Can you work these out from the model? Positions are in its coordinate system, mm. A direction names the side the tool comes from. Coordinates: 2 decimals unless noted, no trailing zeros. Order: outer loops, then holes, each group sorted by start corner. A loop starts at its lowest first (then second) coordinate and runs counter-clockwise, first axis right, second up. Notation, with made-up numbers: (85.25, 10.25) -> (128.25, 10.25) arc R28 cw to (128.25, 38.25) -> close; hole circle Ø9 at (-21, 68.5). An arc over 180 degrees is marked (long way). Write item = value, one per line. Start each with the question number.
from build123d import *

# Parameters (mm, degrees)
BOSS_EXTRUDE1_DEPTH            = 9.525
CUT_EXTRUDE2_DEPTH             = 4
M3_CLEARANCE_HOLE1_D           = 3.2
M3_CLEARANCE_HOLE1_CSINK_D     = 3.45
M3_CLEARANCE_HOLE1_CSINK_ANGLE = 90
FILLET1_R                      = 1


with BuildPart() as part:
    # Sketch2 → Boss-Extrude1 (new body)
    with BuildSketch(Plane(origin=(0, 0, 0), x_dir=(0, 1, 0), z_dir=(0, 0, 1))):
        with BuildLine():
            Line((-9, 10), (9, 10))
            Line((9, 10), (50.45475081, -78.9))
            ThreePointArc((50.45475081, -78.9), (0, -93.653039883), (-50.45475081, -78.9))
            Line((-50.45475081, -78.9), (-9, 10))
        make_face()
    extrude(amount=BOSS_EXTRUDE1_DEPTH)

    # Sketch3 → Cut-Extrude2 (cut)
    with BuildSketch(Plane(origin=(0, 0, 0), x_dir=(1, 0, 0), z_dir=(0, 0, -1))):
        with BuildLine():
            Line((-10, -4.5), (-10, 4.5))
            Line((-10, 4.5), (0, 4.5))
            ThreePointArc((0, 4.5), (4.5, 0), (0, -4.5))
            Line((0, -4.5), (-10, -4.5))
        make_face()
    extrude(amount=-CUT_EXTRUDE2_DEPTH, mode=Mode.SUBTRACT)

    # M3 Clearance Hole1 (through all)
    with Locations(Plane(origin=(0, 0, 9.525), x_dir=(0, -1, 0), z_dir=(0, 0, 1))):
        with Locations((0, 0), (0, -4)):
            CounterSinkHole(M3_CLEARANCE_HOLE1_D / 2, M3_CLEARANCE_HOLE1_CSINK_D / 2, counter_sink_angle=M3_CLEARANCE_HOLE1_CSINK_ANGLE)

    # Fillet1
    fillet1_edges = [part.edges().sort_by_distance(p)[0] for p in [
        (-10, 4.5, 2),
        (-10, -4.5, 2),
        (-10, -9, 4.7625),
        (-10, 9, 4.7625),
        (78.9, 50.45475081, 4.7625),
        (78.9, -50.45475081, 4.7625),
    ]]
    fillet(fillet1_edges, radius=FILLET1_R)


solid = part.part
(1) If I drill on L1, parallel to Y at x = 0, z = 6.05; L2, parallel to Y at x = -4, z = 8.05; L3, parallel to X at y = -41, z = 2, over which ranges is the centre line in solid material (lowest first)? Write a range as from..to.
(2) Imagine slicing it at C-C (z = 2.5). Write out the boundary of the cut face in (x, y).
(3) Imagine slicing it at A-A (y = 0). Write out the boundary of the cut face in (x, z) (3 decimals).
(4) For faces 1 (the face through (-2.6, 1.1, 4)), 2 (the face through (33.73, 29.39, 4.7)), which set-ups out of +Z, -Z, +X, -X, +Y, -Y let a thin tool reach every point of the face, with its end or its side?
(5) Imagine slicing it at D-D (x = 39). Write out the boundary of the cut face in (y, z) (3 decimals), plus the area to 3 significant figures.
(6) For P1, Ø2, axis at y = -36, z = 4, coming from the -X side; P2, Ø1.2, axis at x = -6, z = 1, coming from the +Y side (3 decimals); P3, Ø1.2, axis at x = -6, z = 1.5, coming from the -Y side (3 decimals), each with a flat end and sliding along its axis, tell me the tip position at first contact or that it passes through.
(7) Thinking about a two-plate mould opening in Y: for faces 3 (the face through (93.65, 0.73, 4.7)), 4 (the face through (-0.97, -1.27, 6.66)), 5 (the face through (53, 1, 9.525)), which applies, +Y half, -Y half, draft (parallel to the pull), parting line (faces both ways), or undercut?
(8) Imagine slicing it at B-B (x = -4). Write out the boundary of the cut face in (y, z) (3 decimals), plus the area to 3 significant figures.
Result set:
q1.L1 = -13.66..-1.6, 1.6..13.66
q1.L2 = -11.8..-1.6, 1.6..11.8
q1.L3 = 58.62..84.2
q2.outline = (-10, -8.36) arc R1 ccw to (-9.42, -9.27) -> (78.1, -50.08) arc R1 ccw to (79.37, -49.71) arc R93.65 ccw to (79.37, 49.71) arc R1 ccw to (78.1, 50.08) -> (-9.42, 9.27) arc R1 ccw to (-10, 8.36) -> (-10, 5.5) arc R1 ccw to (-9, 4.5) -> (0, 4.5) arc R4.5 cw to (0, -4.5) -> (-9, -4.5) arc R1 ccw to (-10, -5.5) -> close
q3.outline = (-10, 4) -> (-5.6, 4) -> (-5.6, 9.4) -> (-5.725, 9.525) -> (-10, 9.525) -> close; (-2.4, 4) -> (-1.6, 4) -> (-1.6, 9.4) -> (-1.725, 9.525) -> (-2.275, 9.525) -> (-2.4, 9.4) -> close; (1.6, 4) -> (4.5, 4) -> (4.5, 0) -> (93.653, 0) -> (93.653, 9.525) -> (1.725, 9.525) -> (1.6, 9.4) -> close
q4.face_1 = -Z, -X
q4.face_2 = +Z, -Z, -X, +Y
q5.outline = (-31.849, 0) -> (31.849, 0) -> (31.849, 9.525) -> (-31.849, 9.525) -> close
q5.area = 607 mm2
q6.P1 = 45.76
q6.P2 = 11.145
q6.P3 = -11.145
q7.face_3 = parting line
q7.face_4 = undercut
q7.face_5 = draft
q8.outline = (-11.798, 0) -> (-4.5, 0) -> (-4.5, 4) -> (-1.6, 4) -> (-1.6, 9.4) -> (-1.725, 9.525) -> (-11.798, 9.525) -> close; (1.6, 4) -> (4.5, 4) -> (4.5, 0) -> (11.798, 0) -> (11.798, 9.525) -> (1.725, 9.525) -> (1.6, 9.4) -> close
q8.area = 171 mm2
